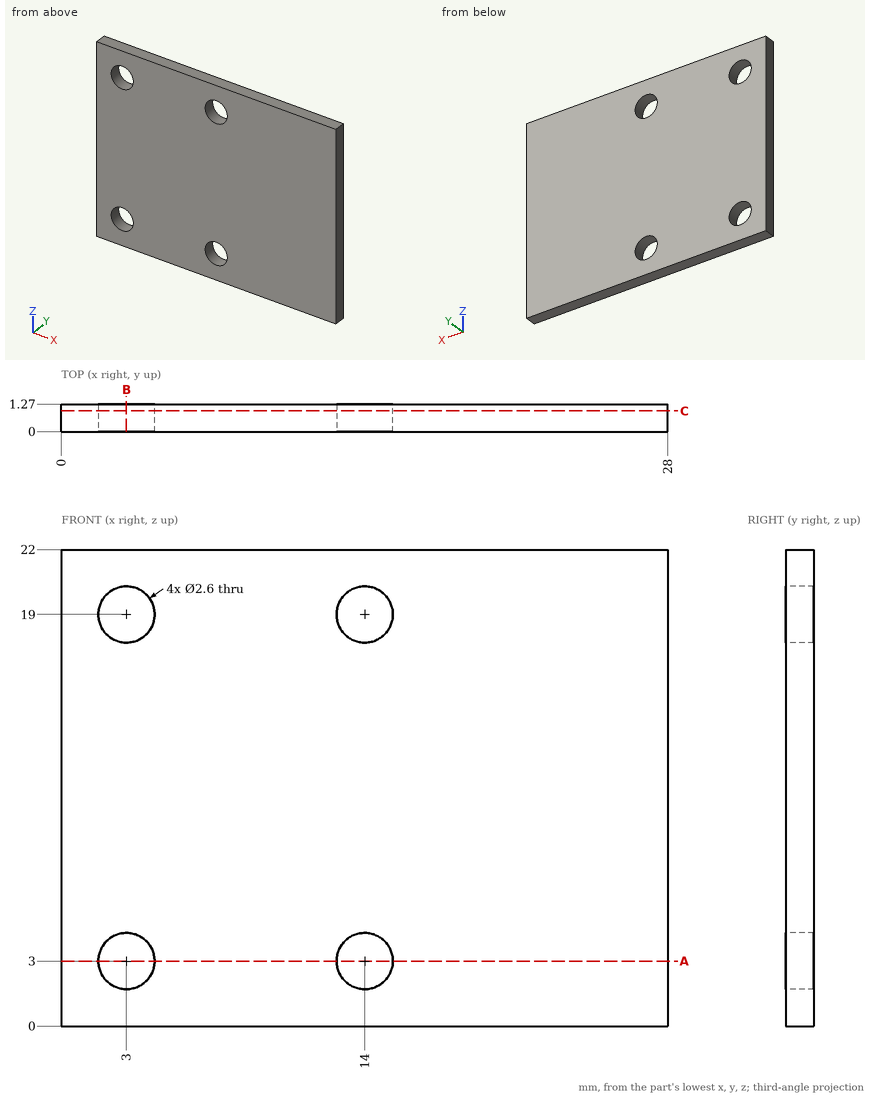
Source: three-view drawing plus pictorial views. Frame: mm from the lowest corner of the part. Round coordinates to 2 decimals unless told otherwise and drop trailing zeros. Order: outer loops, then holes, each group sorted by start corner. A loop starts at its lowest first (then second) coordinate and runs counter-clockwise, first axis right, second up. Notation, with made-up numbers: (8, -28) -> (59, -28) arc R20 ccw to (59, -5) -> close; hole circle Ø1 at (39.25, -40). An arc over 180 degrees is marked (long way). Use one line per item in the form item = value. Start each with the question number.
1. Line query: probe 1 along X at (y, z) = (0.6, 3); probe 2 along Z at (x, y) = (3, 0.5); probe 3 along Z at (x, y) = (3.5, 0.2). Output: solid intervals per line, ascending.
2. Cut plane A-A (z = 3). Return the cut outline in (x, y), then the cut area to 3 significant figures.
3. Cut plane B-B (x = 3). Return the cut outline in (y, z), then the cut area to 3 significant figures.
4. Cut plane C-C (y = 0.95). Return the cut outline in (x, z), then the cut area to 3 significant figures.
Solution:
q1.probe_1 = 0 to 1.7, 4.3 to 12.7, 15.3 to 28
q1.probe_2 = 0 to 1.7, 4.3 to 17.7, 20.3 to 22
q1.probe_3 = 0 to 1.8, 4.2 to 17.8, 20.2 to 22
q2.outline = (0, 0) -> (1.7, 0) -> (1.7, 1.27) -> (0, 1.27) -> close; (4.3, 0) -> (12.7, 0) -> (12.7, 1.27) -> (4.3, 1.27) -> close; (15.3, 0) -> (28, 0) -> (28, 1.27) -> (15.3, 1.27) -> close
q2.area = 29.0 mm^2
q3.outline = (0, 0) -> (1.27, 0) -> (1.27, 1.7) -> (0, 1.7) -> close; (0, 4.3) -> (1.27, 4.3) -> (1.27, 17.7) -> (0, 17.7) -> close; (0, 20.3) -> (1.27, 20.3) -> (1.27, 22) -> (0, 22) -> close
q3.area = 21.3 mm^2
q4.outline = (0, 0) -> (28, 0) -> (28, 22) -> (0, 22) -> close; hole circle Ø2.6 at (3, 3); hole circle Ø2.6 at (3, 19); hole circle Ø2.6 at (14, 3); hole circle Ø2.6 at (14, 19)
q4.area = 595 mm^2
